```python
from build123d import *

# Parameters (mm, degrees)
SKETCH_W        = 20
SKETCH_H        = 10
PAD_DEPTH       = 10
POCKET_DEPTH    = 7
SKETCH002_R     = 3
POCKET001_DEPTH = 7
SKETCH003_R     = 1.5
POCKET002_DEPTH = 5
FILLET_R        = 3


with BuildPart() as part:
    # Sketch → Pad (new body)
    with BuildSketch(Plane.XY):
        Rectangle(SKETCH_W, SKETCH_H)
    extrude(amount=PAD_DEPTH)

    # Sketch001 (on Face1 of Pad) → Pocket (cut)
    with BuildSketch(Plane.XZ.offset(5)):
        with BuildLine():
            Line((-10, 4), (-10, 6))
            Line((-10, 6), (-7, 6))
            ThreePointArc((-7, 4), (-3.267949, 5), (-7, 6))
            Line((-10, 4), (-7, 4))
        make_face()
    pocket = extrude(amount=-POCKET_DEPTH, mode=Mode.SUBTRACT)

    # Sketch002 (on Face1 of Pocket) → Pocket001 (cut)
    with BuildSketch(Plane.XZ.offset(5)):
        with Locations((-5.267949, 5)):
            Circle(SKETCH002_R)
    pocket001 = extrude(amount=-POCKET001_DEPTH, mode=Mode.SUBTRACT)

    # Sketch003 (on Face9 of Pocket001) → Pocket002 (cut)
    with BuildSketch(Plane.XZ.offset(-2)):
        with Locations((-5.267949, 5)):
            Circle(SKETCH003_R)
    pocket002 = extrude(amount=-POCKET002_DEPTH, mode=Mode.SUBTRACT)

    # Mirrored: Pocket, Pocket001, Pocket002 across Sketch001 V_Axis
    add(pocket.mirror(Plane(origin=(0, -5, 0), x_dir=(0, -1, 0), z_dir=(1, 0, 0))), mode=Mode.SUBTRACT)
    add(pocket001.mirror(Plane(origin=(0, -5, 0), x_dir=(0, -1, 0), z_dir=(1, 0, 0))), mode=Mode.SUBTRACT)
    add(pocket002.mirror(Plane(origin=(0, -5, 0), x_dir=(0, -1, 0), z_dir=(1, 0, 0))), mode=Mode.SUBTRACT)

    # Fillet
    fillet_edges = [part.edges().sort_by_distance(p)[0] for p in [
        (-10, 0, 10),
        (-10, 0, 0),
        (10, 0, 10),
        (10, 0, 0),
    ]]
    fillet(fillet_edges, radius=FILLET_R)


solid = part.part
```
Source: CAD feature listing. Evaluate the final solid. Frame: model axes, mm. A direction names the side the tool comes from. Coordinates: 2 decimals unless noted, no trailing zeros. Loops run counter-clockwise (first coordinate to the right, second up) from the corner with the lowest first, then second, coordinate; pieces in that order, holes last. Notation, with made-up numbers: M 79.5,88 L 99.5,88 A20 ccw 99.5,98 Z; hole C 19,44.5 d4. An arc over 180 degrees is marked long. Put each result on its own line as item: value. Start each with the question number.
1) Pull-direction query (Z, two-part tool) for faces 6 (the face through (-9, -2, 4)), 7 (the face through (0, 0, 0)), 8 (the face through (-10, 2.2, 5)), 9 (the face through (-9.14, 0.07, 9.1)); classes: pulls with the +Z half, pulls with the -Z half, needs draft (parallel to the pull), parting line crosses it, or undercut.
2) Cut plane A-A on z = 5. Return the cut outline in (x, y).
3) Cut plane B-B on y = 3. Return the cut outline in (x, z), then the cut area to 3 significant figures.
4) Reachability of faces 1 (the face through (2.27, -1.55, 4.88)), 2 (the face through (9.1, 0.07, 0.86)), 3 (the face through (9, -2, 4)), 4 (the face through (-9, -2, 6)), 5 (the face through (0, 5, 5)) from +Z, -Z, +X, -X, +Y, -Y: full face, straight path, thin tool, end or side. Return the list, or none.
5) Cut plane C-C on x = -3.25. Return the cut outline in (y, z), then the cut area to 3 significant figures.
6) Ray query, L1, parallel to X at y = -3.75, z = 3.75; L2, parallel to X at y = 1, z = 7.75; L3, parallel to Y at x = 3.5, z = 6.5. Return the intervals inside material, ascending. Write a range as from..to.
7) Cut plane D-D on y = -0.75. Return the cut outline in (x, z).
8) Contact query for flat-ended pins moving along their axis: pin 1 Ø3.5 at (x, z) = (-5.27, 5) entering from -Y; pin 2 Ø1.5 at (x, y) = (9.5, -0.5) entering from +Z; pin 3 Ø2 at (x, y) = (-9, -2) entering from -Z; pin 4 Ø1.8 at (x, z) = (-5.27, 5) entering from +Y. Output: stop coordinate, or through.
The answers:
1. face 6: undercut
1. face 7: pulls with the -Z half
1. face 8: needs draft
1. face 9: pulls with the +Z half
2. outline: M -10,2 L -6.77,2 L -6.77,5 L -10,5 Z; M -3.77,2 L -2.27,2 L -2.27,-5 L 2.27,-5 L 2.27,2 L 3.77,2 L 3.77,5 L -3.77,5 Z; M 6.77,2 L 10,2 L 10,5 L 6.77,5 Z
3. outline: M -10,3 A3 ccw -7,0 L 7,0 A3 ccw 10,3 L 10,7 A3 ccw 7,10 L -7,10 A3 ccw -10,7 Z; hole C -5.27,5 d3; hole C 5.27,5 d3
3. area: 178 mm²
4. face 1: -Y
4. face 2: -Z, +X, +Y, -Y
4. face 3: +X, -Y
4. face 4: -X, -Y
4. face 5: +Z, -Z, +X, -X, +Y
5. outline: M -5,0 L 5,0 L 5,10 L -5,10 L -5,7.22 L 2,7.22 L 2,2.78 L -5,2.78 Z
5. area: 68.9 mm²
6. L1: x = -10..-8, -2.54..2.54, 8..10
6. L2: x = -9.9..-6.47, -4.07..4.07, 6.47..9.9
6. L3: y = 2..5
7. outline: M -10,3 A3 ccw -7,0 L 7,0 A3 ccw 10,3 L 10,4 L 8.1,4 A3 cw long 8.1,6 L 10,6 L 10,7 A3 ccw 7,10 L -7,10 A3 ccw -10,7 L -10,6 L -8.1,6 A3 cw long -8.1,4 L -10,4 Z
8. pin 1: stops at y = 2
8. pin 2: stops at z = 9.44
8. pin 3: stops at z = 0.17
8. pin 4: passes through
